Verification items for the finished model (mm, model axes). A direction names the side the tool comes from. Coordinates: 2 decimals unless noted, no trailing zeros. Order: outer loops, then holes, each group sorted by start corner. A loop starts at its lowest first (then second) coordinate and runs counter-clockwise, first axis right, second up. Notation, with made-up numbers: M -11.5,-27.5 L -3.5,-27.5 A26 ccw -3.5,-2.5 Z; hole C 60.25,-21.5 d7. An arc over 180 degrees is marked long. Write item = value, one per line.
Autodesk Inventor part; units mm, degrees
ref_plane "Work Plane1" through (-57, 11.25, -57) normal (0, 1, 0) x (0, 0, 1)
ref_plane "YZ Plane" through (0, 0, 0) normal (1, 0, 0) x (0, 1, 0)
ref_plane "XZ Plane" through (0, 0, 0) normal (0, 1, 0) x (-1, 0, 0)
sketch "Sketch1" plane through (0, 0, 0) normal (0, 1, 0) x (-1, 0, 0)
  line L0 (53, -54) -> (53, -3)
  line L1 (21.75, 0) -> (11.75, 0)
  line L2 (3, -3) -> (3, -12.5)
  line L3 (3, -12.5) -> (0, -12.5)
  line L4 (0, -12.5) -> (0, -20.5)
  line L5 (0, -20.5) -> (3, -20.5)
  line L6 (0, -28.5) -> (26.5, -28.5) construction
  line L7 (26.5, -28.5) -> (26.5, -57) construction
  line L8 (3, -20.5) -> (3, -28.5)
  line L9 (3, -54) -> (3, -44.5)
  line L10 (3, -44.5) -> (0, -44.5)
  line L11 (0, -44.5) -> (0, -36.5)
  line L12 (0, -36.5) -> (3, -36.5)
  line L13 (3, -36.5) -> (3, -28.5)
  line L14 (3, -3) -> (11.75, -3)
  line L15 (11.75, -3) -> (11.75, 0)
  line L16 (11.75, 0) -> (21.75, 0)
  line L17 (21.75, 0) -> (21.75, -3)
  line L18 (21.75, -3) -> (53, -3)
  line L19 (21.75, -57) -> (11.75, -57)
  line L20 (3, -54) -> (11.75, -54)
  line L21 (11.75, -54) -> (11.75, -57)
  line L22 (21.75, -57) -> (21.75, -54)
  line L23 (21.75, -54) -> (53, -54)
  point P0 (0, 0)
  dimension "d4" = 8
  dimension "d6" = 8.75
  dimension "d7" = 10
extrude "Extrusion1" add sketch "Sketch1" along normal blind 3
sketch "Sketch2" plane through (0, 0, 0) normal (0, -1, 0) x (1, 0, 0)
  line L0 (-53, -54) -> (-53, -3)
  arc A0 (-53, -33.5) -> (-53, -23.5) centre (-53, -28.5) ccw
  line L1 (-53, -33.5) -> (-53, -23.5)
  point P0 (0, 0)
  dimension "d10" = 10
ref_plane "Work Plane1" through (-57, 11.25, -57) normal (0, 1, 0) x (0, 0, 1)
extrude "Extrusion2" cut sketch "Sketch2" against normal up to surface (11.25 mm away)
properties part number "SoporteCircuito" material "Iron, Cast"
Item 1: Sectioned sample at B-B, the plane x = -7.5. Enter the section's corners in (y, z).
Report:
outline = M 0,-54 L 3,-54 L 3,-3 L 0,-3 Z
Item 2: Release check for a two-part mould opening along Z. For faces 6 (the flat face through (-11.75, 1, -2)), 7 (the flat face through (-37, 1, -54)), 8 (the flat face through (-1, 1, -20.5)) record: pulls with the +Z half, pulls with the -Z half, needs draft (parallel to the pull), parting line crosses it, or undercut.
Report:
face_6 = needs draft
face_7 = pulls with the -Z half
face_8 = undercut
Item 3: Sectioned sample at C-C, the plane z = -28.5. Enter the section's corners in (x, y).
Report:
outline = M -48,0 L -3,0 L -3,3 L -48,3 Z
Item 4: Gauge pin test, flat ends, axial feed: pin 1 (1.5 mm diameter, centred on x = -1, y = 1.5, fed in from +Z); pin 2 (0.9 mm diameter, centred on x = -9, y = 1.5, fed in from +Z); pin 3 (1.5 mm diameter, centred on y = 1, z = -55.5, fed in from +X). Record the tip position at first contact, or that the pin passes through.
Report:
pin_1 = -12.5
pin_2 = -3
pin_3 = -11.75
Item 5: Sectioned sample at A-A, the plane y = 0.85. Enter the section's corners in (x, z), then the cut area to 3 significant figures.
Report:
outline = M -53,-54 L -21.75,-54 L -21.75,-57 L -11.75,-57 L -11.75,-54 L -3,-54 L -3,-44.5 L 0,-44.5 L 0,-36.5 L -3,-36.5 L -3,-20.5 L 0,-20.5 L 0,-12.5 L -3,-12.5 L -3,-3 L -11.75,-3 L -11.75,0 L -21.75,0 L -21.75,-3 L -53,-3 L -53,-23.5 A5 cw -53,-33.5 Z
area = 2,620 mm^2
Item 6: Scan lines: L1, parallel to Z at x = -27, y = 0.1; L2, parallel to X at y = 1.1, z = -5; L3, parallel to X at y = 1.6, z = -54.5. Record each from-to range of solid material in increasing order. Write a range as from..to.
Report:
L1 = -54..-3
L2 = -53..-3
L3 = -21.75..-11.75
Item 7: Tool access check on faces 1 (the flat face through (-1, 1, -36.5)), 2 (the flat face through (-2, 1, -44.5)), 3 (the flat face through (-21.75, 1, -56)), 4 (the flat face through (-37, 1, -3)), 5 (the flat face through (-3, 1, -8)). Record the directions out of +Z, -Z, +X, -X, +Y, -Y that give a thin tool (end or side, any length) a straight path to the whole face; none if there is none.
Report:
face_1 = +X, +Y, -Y
face_2 = -Z, +X, +Y, -Y
face_3 = -Z, -X, +Y, -Y
face_4 = +Z, -X, +Y, -Y
face_5 = +Z, +X, +Y, -Y
